The listing builds one solid part. Answer for the finished solid, in the listing's coordinates (mm). Face numbers are marked on the shaded views. A direction names the side the tool comes from. Coordinates: 2 decimals unless noted, no trailing zeros. Order: outer loops, then holes, each group sorted by start corner. A loop starts at its lowest first (then second) coordinate and runs counter-clockwise, first axis right, second up. Notation, with made-up numbers: (55, 67) - (70, 67) arc R31 ccw to (70, 106) - close; hole circle Ø8 at (28, 14). An arc over 180 degrees is marked (long way). Use one line per item in the form item = value. Start each with the question number.
Item 1: Consider line 1 along Y through (x, z) = (34, 5); line 2 along Z through (x, y) = (14.5, -7); line 3 along Y through (x, z) = (36, -14.5). Determine where each line is inside the solid, lowest interval first. Write a range as [from, to].
Item 2: Each of these flat-tipped pins is pushed along its axis until it touches: pin 1 Ø11.5 at (x, z) = (59, -13.5) entering from +Y; pin 2 Ø1.5 at (x, z) = (18, 14.5) entering from +Y; pin 3 Ø6 at (y, z) = (64.5, 13) entering from +X. Where does it stop, or does it pass through?
Item 3: Section A-A, the plane z = -9 is taken. Write down the section's boundary in (x, y), and give its area (3 significant figures).
Item 4: Section B-B, the plane y = 54 is taken. Write down the section's boundary in (x, z).
Item 5: A tool of negligible diameter and unlimited length cuts with its end or side. For the marked faces 1, 2 and 3, from which of +Z, -Z, +X, -X, +Y, -Y can it reach the whole face along a straight path? Write none if from no direction.
from build123d import *

# Parameters (mm, degrees)
F1_DEPTH = 20.55
F3_DEPTH = 38
F4_W     = 202.725
F4_H     = 2
F5_DEPTH = 58.551


with BuildPart() as f1:
    # F0 (on Top) → F1 (new body)
    with BuildSketch(Plane.XY):
        Polygon((-63.3625, 110.8625), (-101.3625, 110.8625), (-101.3625, -110.8625), (101.3625, -110.8625), (101.3625, -53.8625), (-63.3625, -53.8625), align=None)
    extrude(amount=F1_DEPTH)

    # F2 (on face) → F3 (join)
    with BuildSketch(Plane(origin=(0, 0, 0), x_dir=(1, 0, 0), z_dir=(0, 0, -1))):
        Polygon((101.3625, -31.8625), (101.3625, 110.8625), (-101.3625, 110.8625), (-101.3625, -110.8625), (22.3625, -110.8625), (22.3625, -31.8625), align=None)
    extrude(amount=F3_DEPTH)

    # F4 (on face) → F5 (cut, through all)
    with BuildSketch(Plane.XY.offset(20.55)):
        with Locations((0, -109.8625)):
            Rectangle(F4_W, F4_H)
    extrude(amount=-F5_DEPTH, mode=Mode.SUBTRACT)


solid = f1.part
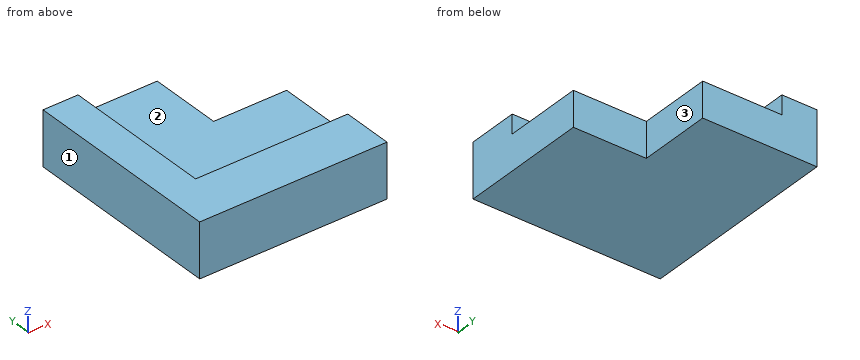
Response:
q1.line_1 = [-108.86, -53.86]
q1.line_2 = [-38, 0]
q1.line_3 = [-108.86, 31.86]
q2.pin_1 = 31.86
q2.pin_2 = -53.86
q2.pin_3 = -63.36
q3.outline = (-101.36, -108.86) - (101.36, -108.86) - (101.36, 31.86) - (22.36, 31.86) - (22.36, 110.86) - (-101.36, 110.86) - close
q3.area = 38,300 mm2
q4.outline = (-101.36, -38) - (22.36, -38) - (22.36, 0) - (-63.36, 0) - (-63.36, 20.55) - (-101.36, 20.55) - close
q5.face_1 = +Z, -Z, -X, +Y, -Y
q5.face_2 = +Z, +X, +Y
q5.face_3 = +Z, -Z, +X, +Y
